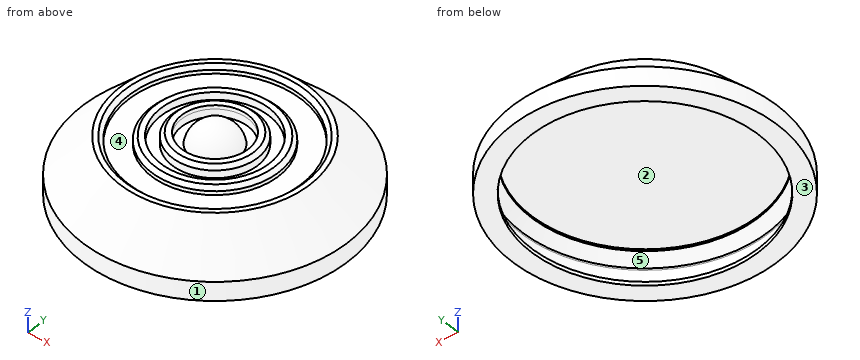
from build123d import *

# Parameters (mm, degrees)
F0_R         = 35
F1_DEPTH     = 15
F2_SIZE      = 10
F4_R         = 22.75
F4_R_2       = 16.75
F5_DEPTH     = 2
F4_R_3       = 14.25
F4_R_4       = 11.25
F6_DEPTH     = 2
F4_R_5       = 8.75
F7_DEPTH     = 2
F8_DEPTH     = 1
F12_R        = 30
F13_DEPTH    = 9.5
F15_R        = 32.5
F16_DEPTH    = 5
F17_S5_R     = 32.5
F17_T6_DEPTH = 48


# Not quite as in the source:
# - a fillet or chamfer that OpenCascade refuses, or shapes differently, is made with other operations: its cross-section is extruded or revolved along the edge and cut away or added


with BuildPart() as f1:
    # F0 (on Top) → F1 (new body)
    with BuildSketch(Plane.XY):
        Circle(F0_R)
    extrude(amount=F1_DEPTH)

    # F2
    f2_edges = [f1.edges().sort_by_distance(p)[0] for p in [
        (-35, 0, 15),
    ]]
    chamfer(f2_edges, length=F2_SIZE)

    # F4 (on offset) → F5 (cut)
    with BuildSketch(Plane.XY.offset(15)):
        Circle(F4_R)
        Circle(F4_R_2, mode=Mode.SUBTRACT)
    extrude(amount=-F5_DEPTH, mode=Mode.SUBTRACT)

    # F4 (on offset) → F6 (cut)
    with BuildSketch(Plane.XY.offset(15)):
        Circle(F4_R_3)
        Circle(F4_R_4, mode=Mode.SUBTRACT)
    extrude(amount=-F6_DEPTH, mode=Mode.SUBTRACT)

    # F4 (on offset) → F7 (cut)
    with BuildSketch(Plane.XY.offset(15)):
        Circle(F4_R_5)
    extrude(amount=-F7_DEPTH, mode=Mode.SUBTRACT)

    # F4 (on offset) → F8 (join)
    with BuildSketch(Plane.XY.offset(15)):
        Circle(F4_R_4)
        Circle(F4_R_5, mode=Mode.SUBTRACT)
    extrude(amount=F8_DEPTH)

    # F9 (on Front) → F10 (revolve)
    with BuildSketch(Plane.XZ):
        with BuildLine():
            Line((0, 12), (0, 5.5))
            ThreePointArc((0, 5.5), (4.5961940777, 7.4038059223), (6.5, 12))
            Line((6.5, 12), (0, 12))
        make_face()
        with BuildLine():
            Line((0, 18.5), (0, 12))
            Line((0, 12), (6.5, 12))
            ThreePointArc((6.5, 12), (4.5961940777, 16.5961940777), (0, 18.5))
        make_face()
    revolve(axis=Axis((0, 0, 6), (0, 0, 1)))

    # F11: chamfer of 1 on 3 edges, made by hand

    # F11_s1 → F11_t2 (revolve, cut)
    with BuildSketch(Plane.XZ):
        Polygon((23.75, 15), (22.75, 14), (22.75, 15), align=None)
    revolve(axis=Axis((0, 0, 15), (0, 0, 1)), mode=Mode.SUBTRACT)

    # F11_s3 → F11_t4 (revolve, cut)
    with BuildSketch(Plane.XZ):
        Polygon((16.75, 14), (15.75, 15), (16.75, 15), align=None)
    revolve(axis=Axis((0, 0, 15), (0, 0, 1)), mode=Mode.SUBTRACT)

    # F11_s5 → F11_t6 (revolve, cut)
    with BuildSketch(Plane.XZ):
        Polygon((11.25, 15), (10.25, 16), (11.25, 16), align=None)
    revolve(axis=Axis((0, 0, 16), (0, 0, 1)), mode=Mode.SUBTRACT)

    # F12 (on Top) → F13 (cut)
    with BuildSketch(Plane.XY):
        Circle(F12_R)
    extrude(amount=F13_DEPTH, mode=Mode.SUBTRACT)

    # F15 (on offset) → F16 (cut)
    with BuildSketch(Plane.XY.offset(1)):
        Circle(F15_R)
    extrude(amount=F16_DEPTH, mode=Mode.SUBTRACT)

    # F17: chamfer of 3 on 1 edges, made by hand


with BuildPart() as f17_tool2:
    # F17_s3 → F17_t4 (revolve)
    with BuildSketch(Plane.XZ):
        Polygon((33, 6), (30, 9), (30, 6), align=None)
    revolve(axis=Axis((0, 0, 6), (0, 0, -1)))

    # F17_s5 → F17_t6 (intersect, symmetric)
    with BuildSketch(Plane.XY.offset(7.5)):
        Circle(F17_S5_R)
    extrude(amount=F17_T6_DEPTH, both=True, mode=Mode.INTERSECT)


with BuildPart() as f1_1:
    add(f1.part)

    # F17_t1: cut F17_tool2
    add(f17_tool2.part, mode=Mode.SUBTRACT)


solid = f1_1.part
Work out the finished part from the listing and answer in its coordinate system (mm). Face numbers are marked on the shaded views. A direction names the side the tool comes from. Coordinates: 2 decimals unless noted, no trailing zeros. Loops run counter-clockwise (first coordinate to the right, second up) from the corner with the lowest first, then second, coordinate; pieces in that order, holes last. Notation, with made-up numbers: (69, 45.25) -> (109, 45.25) arc R12 cw to (109, 65.25) -> close; hole circle Ø4 at (32, 56). An arc over 180 degrees is marked (long way). Answer as CSV lines item,"result".
1) For the marked faces 4 and 5, determine the directions among +Z, -Z, +X, -X, +Y, -Y from which every point of the face is accessible in a straight line to the end or side of a thin tool.
A:
face 4,"+Z"
face 5,"none"
2) Flat-ended cylindrical pins translate along their axes: pin 1 (4 mm diameter, centred on x = -5.5, y = -24, fed in from -Z); pin 2 (23 mm diameter, centred on x = -2.5, y = 11, fed in from +Z); pin 3 (1 mm diameter, centred on y = 6.5, z = 6.5, fed in from -X); pin 4 (1 mm diameter, centred on y = 23.5, z = 3.5, fed in from +X). Find the tip coordinate at first contact, or state that the pin passes through.
A:
pin 1,"stops at z = 9.5"
pin 2,"stops at z = 18.5"
pin 3,"stops at x = -33.38"
pin 4,"stops at x = 26.38"
3) The part is cut by section B-B (z = 11.5). Give the vertices of the cut face in (x, y).
A:
outline,"circle Ø57 at (0, 0)"
4) The part is cut by section A-A (z = 4). Give the vertices of the cut face in (x, y), and give its area (3 significant figures).
A:
outline,"circle Ø70 at (0, 0); hole circle Ø65 at (0, 0)"
area,"530 mm²"
5) Straight lines are drawn through the part: probe 1 along Y at (x, z) = (0, 15.6); probe 2 along Z at (x, y) = (-3.5, -6); probe 3 along Y at (x, z) = (-9.5, 6). For each, find the intervals that lie inside material, in ascending order.
A:
probe 1,"y = -10.65 to -8.75, -5.41 to 5.41, 8.75 to 10.65"
probe 2,"z = 9.5 to 13"
probe 3,"y = -32.65 to -31.08, 31.08 to 32.65"
6) For a pull along X with two mould halves and no side action, classify the marked faces 1, 2 and 3 as released by +X, released by -X, zero draft, split by the parting line, or undercut.
A:
face 1,"split by the parting line"
face 2,"undercut"
face 3,"zero draft"
